The model under review builds one solid part; all positions refer to its coordinate system, in mm. Coordinates: 2 decimals unless noted, no trailing zeros. Loops run counter-clockwise (first coordinate to the right, second up) from the corner with the lowest first, then second, coordinate; pieces in that order, holes last. Notation, with made-up numbers: M -8,32.5 L 13,32.5 A21 cw 13,45.5 Z; hole C -25.5,60.5 d5. An arc over 180 degrees is marked long. One line per item, written item: value.
Autodesk Inventor part; units mm, degrees
ref_plane "YZ Plane" through (0, 0, 0) normal (1, 0, 0) x (0, 1, 0)
ref_plane "XZ Plane" through (0, 0, 0) normal (0, 1, 0) x (-1, 0, 0)
ref_plane "XY Plane" through (0, 0, 0) normal (0, 0, 1) x (1, 0, 0)
sketch "Sketch1" plane through (0, 0, 0) normal (0, 1, 0) x (-1, 0, 0)
  line L0 (0, 0) -> (-50, 0)
  line L1 (-50, 0) -> (-50, -50)
  line L2 (-50, -50) -> (0, -50)
  line L3 (0, -50) -> (0, 0)
  point P0 (-7.5, -7.5)
  point P1 (-7.5, -42.5)
  point P2 (-42.5, -42.5)
  point P3 (-42.5, -7.5)
  dimension "d0" = 50
  dimension "d1" = 50
  dimension "d2" = 35
  dimension "d3" = 7.5
  dimension "d4" = 35
  dimension "d5" = 35
  dimension "d6" = 7.5
  dimension "d7" = 7.5
  dimension "d23" = 35
  dimension "d24" = 7.5
extrude "Extrusion1" add sketch "Sketch1" along normal blind 5
sketch "Sketch2" plane through (0, 5, 0) normal (0, 1, 0) x (1, 0, 0)
  line L0 (50, 50) -> (0, 50)
  line L1 (0, 50) -> (0, 0)
  point P0 (7.5, 7.5)
  point P1 (7.5, 42.5)
  point P2 (42.5, 42.5)
  point P3 (42.5, 7.5)
  dimension "d10" = 35
  dimension "d11" = 35
  dimension "d12" = 35
  dimension "d13" = 7.5
  dimension "d14" = 7.5
  dimension "d15" = 7.5
  dimension "d25" = 35
  dimension "d26" = 7.5
hole "Hole1" at (7.5, 5, -7.5) at (7.5, 5, -42.5) at (42.5, 5, -42.5) at (42.5, 5, -7.5) direction (0, -1, 0) diameter 3.4587 end through all
sketch "Sketch3" plane through (0, 5, 0) normal (0, 1, 0) x (1, 0, 0)
  line L0 (0, 0) -> (50, 0)
  line L1 (0, 50) -> (0, 0)
  point P0 (25, 25)
  dimension "d27" = 25
  dimension "d28" = 25
hole "Hole2" at (25, 5, -25) direction (0, -1, 0) diameter 3 end through all
equation "\"d21\" = Thickness"
equation "\"BendRadius\" = Thickness"
equation "\"BendReliefWidth\" = Thickness"
equation "\"BendReliefDepth\" = 0.5 * Thickness"
equation "\"CornerReliefSize\" = 4 * Thickness"
equation "\"MinimumRemnant\" = 2 * Thickness"
equation "\"TransitionRadius\" = BendRadius"
equation "\"JacobiRadiusSize\" = BendRadius"
equation "\"GapSize\" = Thickness"
properties part number "Bottom link plate"
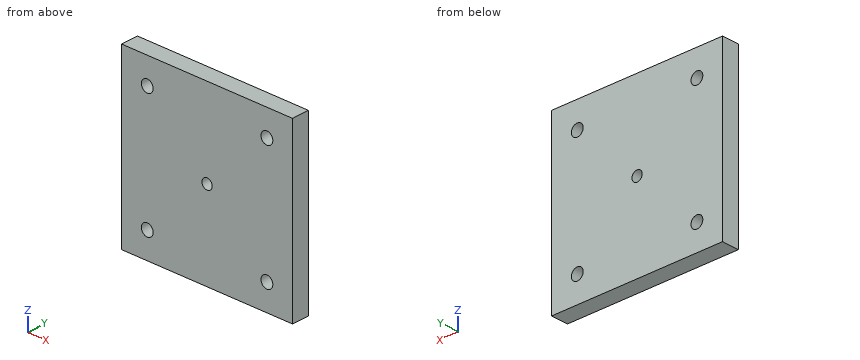
(1) Insertion check: pin 1 Ø3 at (x, z) = (7.5, -7.5) entering from +Y. The pin has a flat end and moves straight along its axis. Give the tip position at first contact, or say it passes through.
Checks:
pin 1: through
(2) Add section D-D on x = 25. State the section outline as (y, z) points, then the cut area to 3 significant figures.
Checks:
outline: M 0,-50 L 5,-50 L 5,-26.5 L 0,-26.5 Z; M 0,-23.5 L 5,-23.5 L 5,0 L 0,0 Z
area: 235 mm^2
(3) To check wall thickness, follow L1, parallel to X at y = 1.65, z = -42.5; L2, parallel to Z at x = 7.5, y = 1.55; L3, parallel to X at y = 4.45, z = -8.5. State the ranges of each line that lie inside material, in increasing order. Write a range as [from, to].
Checks:
L1: [0, 5.77], [9.23, 40.77], [44.23, 50]
L2: [-50, -44.23], [-40.77, -9.23], [-5.77, 0]
L3: [0, 6.09], [8.91, 41.09], [43.91, 50]
(4) Add section C-C on y = 2.6. State the section outline as (x, z) points, then the cut area to 3 significant figures.
Checks:
outline: M 0,-50 L 50,-50 L 50,0 L 0,0 Z; hole C 7.5,-42.5 d3.46; hole C 7.5,-7.5 d3.46; hole C 25,-25 d3; hole C 42.5,-42.5 d3.46; hole C 42.5,-7.5 d3.46
area: 2,460 mm^2
(5) Add section B-B on x = 42.5. State the section outline as (y, z) points, then the cut area to 3 significant figures.
Checks:
outline: M 0,-50 L 5,-50 L 5,-44.23 L 0,-44.23 Z; M 0,-40.77 L 5,-40.77 L 5,-9.23 L 0,-9.23 Z; M 0,-5.77 L 5,-5.77 L 5,0 L 0,0 Z
area: 215 mm^2
(6) Add section A-A on z = -42.5. State the section outline as (x, y) points.
Checks:
outline: M 0,0 L 5.77,0 L 5.77,5 L 0,5 Z; M 9.23,0 L 40.77,0 L 40.77,5 L 9.23,5 Z; M 44.23,0 L 50,0 L 50,5 L 44.23,5 Z
